```python
from build123d import *

# Parameters (mm, degrees)
F0_R     = 10
F1_DEPTH = 700
F2_R     = 9.75
F3_DEPTH = 2
F4_R     = 10
F4_R_2   = 9.75
F5_DEPTH = 15
F6_R     = 9.75
F7_DEPTH = 2
F8_R     = 10
F8_R_2   = 9.75
F9_DEPTH = 15


with BuildPart() as f1:
    # F0 (on Top) → F1 (new body)
    with BuildSketch(Plane.XY):
        Circle(F0_R)
    extrude(amount=F1_DEPTH)

    # F2 (on face) → F3 (join)
    with BuildSketch(Plane(origin=(0, 0, 0), x_dir=(1, 0, 0), z_dir=(0, 0, -1))):
        Circle(F2_R)
    extrude(amount=F3_DEPTH)

    # F4 (on face) → F5 (join)
    with BuildSketch(Plane(origin=(0, 0, -2), x_dir=(1, 0, 0), z_dir=(0, 0, -1))):
        Circle(F4_R)
        Circle(F4_R_2, mode=Mode.SUBTRACT)
        Circle(F4_R_2)
    extrude(amount=F5_DEPTH)

    # F6 (on face) → F7 (join)
    with BuildSketch(Plane.XY.offset(700)):
        Circle(F6_R)
    extrude(amount=F7_DEPTH)

    # F8 (on face) → F9 (join)
    with BuildSketch(Plane.XY.offset(702)):
        Circle(F8_R)
        Circle(F8_R_2, mode=Mode.SUBTRACT)
        Circle(F8_R_2)
    extrude(amount=F9_DEPTH)


solid = f1.part
```
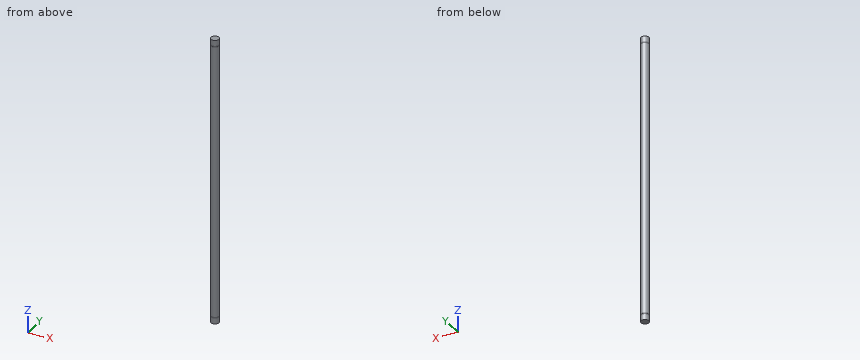
Geometry check sheet. Reference: the model listing, model coordinates, mm. Give positions to 0.01 mm unless a question says otherwise; leave off trailing zeros. Loops run counter-clockwise (first coordinate to the right, second up) from the corner with the lowest first, then second, coordinate; pieces in that order, holes last. Notation, with made-up numbers: M 48,69.25 L 95,69.25 A9 ccw 95,80.25 Z; hole C 16,28 d9. An arc over 180 degrees is marked long. Write item = value, one per line. Start each with the question number.
1. Section check B-B, the plane x = -3.25. Enter the section's corners in (y, z), plus the area to 3 significant figures.
2. Go/stop test with flat-tipped pins: P1, Ø3, axis at x = -6, z = 365, coming from the -Y side; P2, Ø1.5, axis at y = -5.5, z = 419.5, coming from the +X side; P3, Ø8, axis at x = -6, z = 359, coming from the +Y side; P4, Ø6, axis at y = -1, z = 306.5, coming from the +X side. Record where each tip stops, or that it passes through.
3. Section check C-C, the plane z = 530. Enter the section's corners in (x, y), plus the area to 3 significant figures.
4. Thickness scan on probe 1 along Y at (x, z) = (0.5, 353.5); probe 2 along X at (y, z) = (-1, 188); probe 3 along X at (y, z) = (2, 609). Record the ranges inside material, lowest first.
5. Section check A-A, the plane y = -4.5. Enter the section's corners in (x, z), plus the area to 3 significant figures.
Values follow:
q1.outline = M -9.46,-17 L 9.46,-17 L 9.46,-2 L 9.19,-2 L 9.19,0 L 9.46,0 L 9.46,700 L 9.19,700 L 9.19,702 L 9.46,702 L 9.46,717 L -9.46,717 L -9.46,702 L -9.19,702 L -9.19,700 L -9.46,700 L -9.46,0 L -9.19,0 L -9.19,-2 L -9.46,-2 Z
q1.area = 13,900 mm^2
q2.P1 = -8.93
q2.P2 = 8.8
q2.P3 = 9.8
q2.P4 = 10
q3.outline = C 0,0 d20
q3.area = 314 mm^2
q4.probe_1 = -9.99 to 9.99
q4.probe_2 = -9.95 to 9.95
q4.probe_3 = -9.8 to 9.8
q5.outline = M -8.93,-17 L 8.93,-17 L 8.93,-2 L 8.65,-2 L 8.65,0 L 8.93,0 L 8.93,700 L 8.65,700 L 8.65,702 L 8.93,702 L 8.93,717 L -8.93,717 L -8.93,702 L -8.65,702 L -8.65,700 L -8.93,700 L -8.93,0 L -8.65,0 L -8.65,-2 L -8.93,-2 Z
q5.area = 13,100 mm^2
